Here's how the part is built. I have some questions about the finished solid (model axes, mm). A direction names the side the tool comes from. Coordinates: 2 decimals unless noted, no trailing zeros. Write each loop counter-clockwise with the first axis right and the second up, starting at its lowest first coordinate (ties: lowest second). Pieces come first, ordered by that corner, then holes. Notation, with made-up numbers: (64, 28.25) -> (108, 28.25) arc R5 cw to (108, 33.25) -> close; hole circle Ø10 at (37.25, -26). An arc over 180 degrees is marked (long way). Answer in a Markdown table with one row per item. Add a question column.
from build123d import *

# Parameters (mm, degrees)
SKETCH1_W           = 65
SKETCH1_H           = 30
SKETCH1_R           = 1.5
SKETCH1_W_2         = 5
SKETCH1_H_2         = 5
BOSS_EXTRUDE1_DEPTH = 5
FILLET1_R           = 5


with BuildPart() as part:
    # Sketch1 → Boss-Extrude1 (new body)
    with BuildSketch(Plane(origin=(0, 0, 0), x_dir=(0, 0, -1), z_dir=(1, 0, 0))):
        with Locations((32.5, 15)):
            Rectangle(SKETCH1_W, SKETCH1_H)
        with Locations((7.5, 15)):
            Circle(SKETCH1_R, mode=Mode.SUBTRACT)
        with Locations(Location((57.5, 15, 0), (0, 0, 180))):
            Circle(SKETCH1_R, mode=Mode.SUBTRACT)
        with Locations(Location((32.5, 15, 0), (0, 0, 180))):
            Circle(SKETCH1_R, mode=Mode.SUBTRACT)
        with Locations((7.5, 22.5)):
            Rectangle(SKETCH1_W_2, SKETCH1_H_2, mode=Mode.SUBTRACT)
        with Locations((7.5, 7.5)):
            Rectangle(SKETCH1_W_2, SKETCH1_H_2, mode=Mode.SUBTRACT)
        with Locations((57.5, 22.5)):
            Rectangle(SKETCH1_W_2, SKETCH1_H_2, mode=Mode.SUBTRACT)
        with Locations((57.5, 7.5)):
            Rectangle(SKETCH1_W_2, SKETCH1_H_2, mode=Mode.SUBTRACT)
        with Locations((32.5, 22.5)):
            Rectangle(SKETCH1_W_2, SKETCH1_H_2, mode=Mode.SUBTRACT)
        with Locations((32.5, 7.5)):
            Rectangle(SKETCH1_W_2, SKETCH1_H_2, mode=Mode.SUBTRACT)
    extrude(amount=BOSS_EXTRUDE1_DEPTH)

    # Fillet1
    fillet1_edges = [part.edges().sort_by_distance(p)[0] for p in [
        (2.5, 30, 0),
        (2.5, 30, -65),
        (2.5, 0, -65),
        (2.5, 0, 0),
    ]]
    fillet(fillet1_edges, radius=FILLET1_R)


solid = part.part
Q1. Imagine slicing it at B-B on z = -32.5. Please give me the cut outline in (x, y).
Q2. Imagine slicing it at D-D on y = 2.75. Please give me the cut outline in (x, z).
Q3. Imagine slicing it at C-C on x = 3.4. State how many separate pieces and enclosed holes the cut face has, plus the area to 3 significant figures.
Q4. Imagine slicing it at A-A on y = 15. Please give me the cut outline in (x, z).
Q5. I'm going to push flat-ended pins straight in: P1, Ø2, axis at y = 4, z = -7.5, coming from the -X side; P2, Ø2.5, axis at y = 15, z = -57.5, coming from the +X side. Where does each tip first touch, or does it pass through?
Q6. I need wall thicknesses on line 1 (Y direction, x = 1.35, z = -57.5); line 2 (Y direction, x = 1.55, z = -9.5); line 3 (Z direction, x = 4.75, y = 22.25). Which ranges of each line are inside material? Lowest first, please. Write a range as [from, to].
Q7. For faces 1 (the flat face through (2, 22, -60)), 2 (the cylindrical face through (3, 29, -63)), which set-ups out of +Z, -Z, +X, -X, +Y, -Y let a thin tool reach every point of the face, with its end or its side?
Q8. If we mould it in two halves opening along Y, with no side actions, what happens to faces 3 (the flat face through (2, 7, -10)), 4 (the cylindrical face through (3, 2, -1)), 5 (the flat face through (2, 25, -57)), 6 (the flat face through (2, 15, -65))? For each: pulls with the +Y half, pulls with the -Y half, needs draft (parallel to the pull), parting line crosses it, or undercut.
Result sheet:
| question | item | result |
|---|---|---|
| 1 | outline | (0, 0) -> (5, 0) -> (5, 5) -> (0, 5) -> close; (0, 10) -> (5, 10) -> (5, 13.5) -> (0, 13.5) -> close; (0, 16.5) -> (5, 16.5) -> (5, 20) -> (0, 20) -> close; (0, 25) -> (5, 25) -> (5, 30) -> (0, 30) -> close |
| 2 | outline | (0, -64.47) -> (5, -64.47) -> (5, -0.53) -> (0, -0.53) -> close |
| 3 | separate pieces | 1 |
| 3 | enclosed holes | 9 |
| 3 | area | 1,760 mm^2 |
| 4 | outline | (0, -65) -> (5, -65) -> (5, -59) -> (0, -59) -> close; (0, -56) -> (5, -56) -> (5, -34) -> (0, -34) -> close; (0, -31) -> (5, -31) -> (5, -9) -> (0, -9) -> close; (0, -6) -> (5, -6) -> (5, 0) -> (0, 0) -> close |
| 5 | P1 | stops at x = 0 |
| 5 | P2 | passes through |
| 6 | line 1 | y = [0, 5], [10, 13.5], [16.5, 20], [25, 30] |
| 6 | line 2 | y = [0, 5], [10, 20], [25, 30] |
| 6 | line 3 | z = [-65, -60], [-55, -35], [-30, -10], [-5, 0] |
| 7 | face 1 | +X, -X |
| 7 | face 2 | -Z, +X, -X, +Y |
| 8 | face 3 | undercut |
| 8 | face 4 | pulls with the -Y half |
| 8 | face 5 | undercut |
| 8 | face 6 | needs draft |
